Job drawing, mm, ordinate dimensions from the low corner. One solid piece. Round coordinates to 2 decimals unless told otherwise and drop trailing zeros. Write each loop counter-clockwise with the first axis right and the second up, starting at its lowest first coordinate (ties: lowest second). Pieces come first, ordered by that corner, then holes.
1) Saw through at B-B on x = 6.35. Write the cut outline in (y, z) (1 decimal).
2) Drill centre lines: L1, parallel to Z at x = 6.35, y = 69 (1 decimal); L2, parallel to X at y = 29.5, z = 6.5; L3, parallel to X at y = 113, z = 7.25 (1 decimal). Where is each one in solid material? Low to high.
3) Saw through at A-A on z = 6.35. Write the cut outline in (x, y) (1 decimal).
4) Flat gauge pins, fed straight in: pin 1 (1 mm diameter, centred on y = 98, z = 4.5, fed in from +X) (1 decimal); pin 2 (2 mm diameter, centred on x = 3, y = 33.5, fed in from -Z). Where does each tip first touch, or does it go through?
5) Pull direction X, two halves, no side cores. Call the marked faces 1 and 2: +X half, -X half, draft (parallel to the pull), parting line (faces both ways), or undercut.
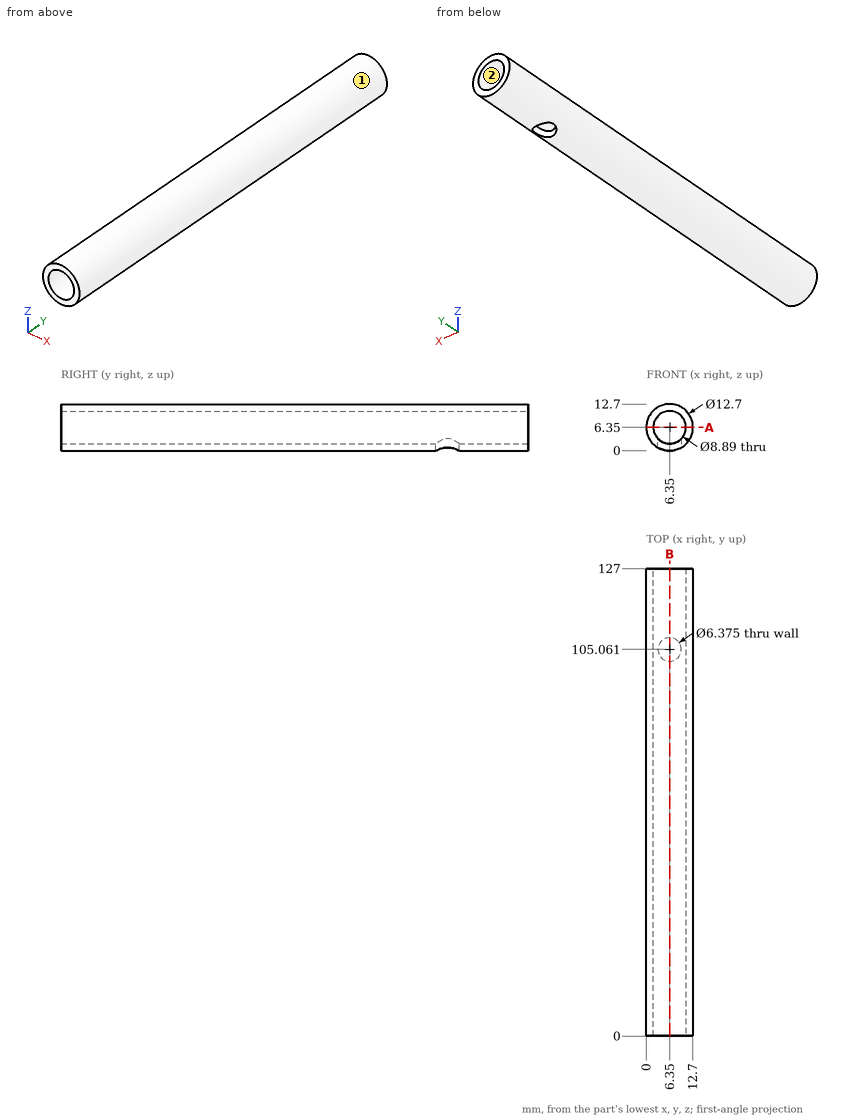
Completed:
1. outline: (0, 0) - (101.9, 0) - (101.9, 1.9) - (0, 1.9) - close; (0, 10.8) - (127, 10.8) - (127, 12.7) - (0, 12.7) - close; (108.2, 0) - (127, 0) - (127, 1.9) - (108.2, 1.9) - close
2. L1: z = 0 to 1.9, 10.8 to 12.7
2. L2: x = 0 to 1.91, 10.79 to 12.7
2. L3: x = 0.1 to 2, 10.7 to 12.6
3. outline: (0, 0) - (1.9, 0) - (1.9, 127) - (0, 127) - close; (10.8, 0) - (12.7, 0) - (12.7, 127) - (10.8, 127) - close
4. pin 1: stops at x = 12.6
4. pin 2: stops at z = 0.45
5. face 1: parting line
5. face 2: undercut
